The listing builds one solid part. Answer for the finished solid, in the listing's coordinates (mm). A direction names the side the tool comes from. Coordinates: 2 decimals unless noted, no trailing zeros. Order: outer loops, then holes, each group sorted by start corner. A loop starts at its lowest first (then second) coordinate and runs counter-clockwise, first axis right, second up. Notation, with made-up numbers: (-27.5, 74.25) - (-19.5, 74.25) arc R23 cw to (-19.5, 89.25) - close; hole circle Ø4 at (22, 67). An arc over 180 degrees is marked (long way). Use a Markdown table: item, result. Add a question column.
Item 1: The part is cut by section C-C, the plane y = -132. Give the vertices of the cut face in (x, z) (3 decimals), then the cut area to 3 significant figures.
Item 2: The mould has two halves that part along Y. Classify faces 3 (the cylindrical face through (-108.33, -112.88, 1.18)), 4 (the cylindrical face through (111.514, -115.941, 1.372)), 5 (the flat face through (-109.13, -118.11, -2.25)), 6 (the flat face through (0.6, -143.1, -9.525)): released by +Y, released by -Y, zero draft, split by the parting line, or undercut.
Item 3: Flat-ended cylindrical pins translate along their axes: P1, Ø3, axis at x = 66.5, z = -5, coming from the +Y side; P2, Ø12, axis at x = -66, y = -120.5, coming from the -Z side (3 decimals); P3, Ø3, axis at x = 65.5, z = -0.5, coming from the +Y side; P4, Ø3, axis at x = 52, z = 3, coming from the -Y side. Find the tip coordinate at first contact, or state that the pin passes through.
Item 4: For faces 1 (the flat face through (109.13, -118.11, -2.25)), 2 (the flat face through (110, -110, 0)), determine the directions among +Z, -Z, +X, -X, +Y, -Y from which every point of the face is accessible in a straight line to the end or side of a thin tool.
Item 5: The part is cut by section D-D, the plane x = 11. Give the vertices of the cut face in (y, z) (3 decimals), then the cut area to 3 significant figures.
Item 6: The part is cut by section A-A, the plane y = -107.5. Give the vertices of the cut face in (x, z) (3 decimals), then the cut area to 3 significant figures.
Item 7: Find the intervals of material crossed by line 1 along X through (y, z) = (-120, 6.75); line 2 along X through (y, z) = (-116, -1.5); line 3 along X through (y, z) = (-104, 1.75), in increasing order.
Autodesk Inventor part; units mm, degrees
ref_plane "YZ Plane" through (0, 0, 0) normal (1, 0, 0) x (0, 1, 0)
ref_plane "XY Plane" through (0, 0, 0) normal (0, 0, 1) x (1, 0, 0)
sketch "Sketch1" plane through (0, 0, 0) normal (0, 0, 1) x (1, 0, 0)
  circle A0 centre (0, 0) radius 142.875
  circle A1 centre (0, 0) radius 149.225
  dimension "innerDiameter" = 285.75
  dimension "outerDiameter" = 298.45
extrude "Extrusion1" add sketch "Sketch1" along normal mid plane 19.05
sketch "Sketch2" plane through (0, 0, 0) normal (0, 0, 1) x (1, 0, 0)
  circle A0 centre (0, 0) radius 142.875 construction
  line L0 (0, 142.875) -> (0, 149.225) construction
  circle A1 centre (0, 0) radius 149.225 construction
  line L1 (0, 142.875) -> (44.45, 142.875)
  line L2 (44.45, 142.875) -> (44.45, 149.225)
  line L3 (44.45, 149.225) -> (19.05, 149.225)
  line L4 (0, 142.875) -> (-44.45, 142.875)
  line L5 (-44.45, 142.875) -> (-44.45, 149.225)
  line L6 (-44.45, 149.225) -> (19.05, 149.225)
  line L7 (371.6693, 35.081) -> (0, 0)
  dimension "halfBaseWidth" = 44.45
  dimension "baseThickness" = 6.35
  dimension "baseHeight" = 0
extrude "Extrusion2" add sketch "Sketch2" along normal mid plane 19.05
sketch "Sketch5" plane through (-44.45, 149.225, 9.525) normal (0, 1, 0) x (1, 0, 0)
  line L0 (0, 19.05) -> (0, 0)
  line L1 (88.9, 19.05) -> (88.9, 0)
  line L2 (0, 0) -> (88.9, 0)
  line L3 (88.9, 0) -> (88.9, 19.05)
  line L4 (88.9, 19.05) -> (0, 19.05)
  line L5 (0, 19.05) -> (0, 0)
  point P0 (44.45, 9.525)
  point P1 (0, 19.05)
extrude "Extrusion3" add sketch "Sketch5" along normal blind 38.1
sketch "Sketch7" plane through (0, 0, 9.525) normal (0, 0, 1) x (1, 0, 0)
  line L0 (-44.45, 142.875) -> (-44.45, 187.325)
  line L1 (-44.45, 187.325) -> (44.45, 187.325)
  line L2 (44.45, 142.875) -> (44.45, 187.325)
  line L3 (0, 187.325) -> (0, 149.1868) construction
  line L4 (-15.875, 169.545) -> (15.875, 169.545)
  line L5 (15.875, 169.545) -> (15.875, 182.245)
  line L6 (15.875, 182.245) -> (-15.875, 182.245)
  line L7 (-15.875, 182.245) -> (-15.875, 169.545)
  line L8 (-15.875, 169.545) -> (15.875, 182.245) construction
  line L9 (15.875, 169.545) -> (-15.875, 182.245) construction
  point P0 (0, 0)
  point P1 (-38.1, 144.2792)
  point P2 (38.1, 144.2792)
  point P3 (0, 175.895)
  dimension "screwHoleWidth" = 31.75
  dimension "screwHoleHeight" = 12.7
  dimension "screwHoleSupportThickness" = 5.08
extrude "Extrusion4" cut sketch "Sketch7" against normal through all
sketch "Sketch6" plane through (-44.45, 187.325, 9.525) normal (0, 1, 0) x (1, 0, 0)
  point P0 (44.45, 9.525)
  point P1 (44.45, 9.525)
hole "Hole2" at (0, 187.325, 0) direction (0, -1, 0) diameter 6.7564 depth 5.08
ref_plane "Work Plane1" through (0, 0, 0) normal (-0.7071, 0.7071, 0) x (0, 0, 1)
ref_plane "Work Plane2" through (0, 0, 0) normal (0.7071, 0.7071, 0) x (0, 0, 1)
sketch "Sketch11" plane through (0, 0, 0) normal (0, 0, 1) x (1, 0, 0)
  arc A0 (-43.0678, 142.875) -> (43.0678, 142.875) centre (0, 0) ccw
  circle A1 centre (0, 0) radius 142.875
  line L0 (-214.9625, 214.9625) -> (217.3313, -217.3313)
  line L1 (-101.0279, 101.0279) -> (-96.5378, 105.518)
  line L2 (-101.0279, 101.0279) -> (-94.6779, 101.0279) construction
  line L3 (-96.5378, 105.518) -> (-114.4983, 123.4785)
  line L4 (-96.5378, 105.518) -> (-71.1378, 105.518) construction
  line L5 (-114.4983, 123.4785) -> (-118.9884, 118.9884)
  line L6 (-118.9884, 118.9884) -> (-101.0279, 101.0279)
  line L7 (-101.0279, 101.0279) -> (-105.518, 96.5378)
  line L8 (-105.518, 96.5378) -> (-123.4785, 114.4983)
  line L9 (-123.4785, 114.4983) -> (-118.9884, 118.9884)
  point P0 (38.1, 144.2792)
  point P1 (-38.1, 144.2792)
  point P2 (-109.9126, 100.9323)
  point P3 (-100.9323, 109.9126)
  dimension "d47" = 6.35
  dimension "d48" = 45
  dimension "d49" = 25.4
  dimension "d50" = 135
extrude "Extrusion7" add sketch "Sketch11" along normal mid plane 19.05 contours A0 L0 L5 L3 | A0 L8 L9 L0
sketch "Sketch12" plane through (-114.4983, 123.4785, -9.525) normal (0.7071, 0.7071, 0) x (-0.7071, 0.7071, 0)
  line L0 (0, 0) -> (0, 19.05)
  line L1 (-19.1852, 19.05) -> (0, 19.05)
  line L2 (-19.1852, 0) -> (-19.1852, 19.05)
  line L3 (0, 0) -> (-19.1852, 0)
  line L4 (-9.5926, 19.05) -> (-9.5926, 0) construction
  line L5 (0, 9.525) -> (-19.1852, 9.525) construction
  point P0 (-168.275, 9.525)
  point P1 (-9.5926, 9.525)
hole "Hole4" at (-107.7153, 116.6955, 0) direction (-0.7071, -0.7071, 0) diameter 5.1054 depth 12.7
pattern_circular "Circular Pattern1" count 4 over 360 about axis through (0, 0, -10) along (0, 0, 1) of "Extrusion7", "Hole4"
sketch "Sketch13" plane through (0, 0, 9.525) normal (0, 0, 1) x (1, 0, 0)
  line L0 (-15.875, 182.245) -> (15.875, 182.245)
  line L1 (-44.45, 187.325) -> (44.45, 187.325)
  line L2 (0, 184.785) -> (8.89, 184.785)
  line L3 (8.89, 184.785) -> (8.89, 182.245)
  line L4 (8.89, 182.245) -> (0, 182.245)
  line L5 (0, 184.785) -> (0, 182.245)
  line L6 (15.875, 182.245) -> (-15.875, 182.245)
  line L7 (0, 184.785) -> (-8.89, 184.785)
  line L8 (-8.89, 184.785) -> (-8.89, 182.245)
  point P0 (0, 0)
  dimension "d63" = 8.89
  dimension "d64" = 2.54
extrude "Extrusion8" cut sketch "Sketch13" against normal through all
split "Split1" plane through (0, 0, 0) removes the side toward (0.7071, 0.7071, 0)
split "Split2" plane through (0, 0, 0) removes the side toward (-0.7071, 0.7071, 0)
equation "\"outerDiameter\" = innerDiameter + 2 * ringThicknessRadius"
equation "\"d7\" = ringWidth"
equation "\"d51\" = ringWidth"
equation "\"ringThicknessRadius\" = 6.35"
properties part number "mountLowerQuarter" material "PET Plastic"
Solution:
| question | item | result |
|---|---|---|
| 1 | outline | (-69.6, -9.525) - (-54.674, -9.525) - (-54.674, 9.525) - (-69.6, 9.525) - close; (54.674, -9.525) - (69.6, -9.525) - (69.6, 9.525) - (54.674, 9.525) - close |
| 1 | area | 569 mm2 |
| 2 | face 3 | undercut |
| 2 | face 4 | undercut |
| 2 | face 5 | released by -Y |
| 2 | face 6 | zero draft |
| 3 | P1 | stops at y = -125.66 |
| 3 | P2 | stops at z = -9.525 |
| 3 | P3 | stops at y = -126.19 |
| 3 | P4 | stops at y = -140.42 |
| 4 | face 1 | +Z, -Z, -Y |
| 4 | face 2 | +Z, -Z, +X, +Y |
| 5 | outline | (-148.819, -9.525) - (-142.451, -9.525) - (-142.451, 9.525) - (-148.819, 9.525) - close |
| 5 | area | 121 mm2 |
| 6 | outline | (-107.5, -9.525) - (-94.112, -9.525) - (-94.112, 9.525) - (-107.5, 9.525) - close; (94.112, -9.525) - (107.5, -9.525) - (107.5, 9.525) - (94.112, 9.525) - close |
| 6 | area | 510 mm2 |
| 7 | line 1 | x = -117.98 to -111.02, -88.7 to -77.55, 77.55 to 88.7, 111.02 to 117.98 |
| 7 | line 2 | x = -116 to -111.33, -93.87 to -83.41, 83.41 to 93.87, 111.33 to 116 |
| 7 | line 3 | x = -104 to -97.97, 97.97 to 104 |
